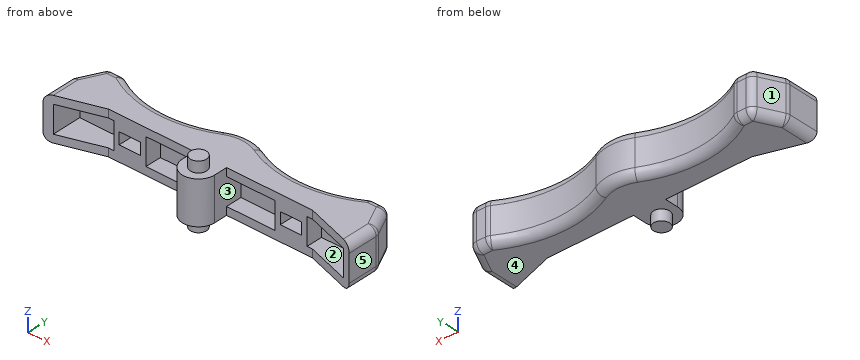
from build123d import *

# Parameters (mm, degrees)
PAD060_DEPTH            = 4
CYLINDER_R              = 1.5
CYLINDER_DEPTH          = 6
SKETCH098_W             = 9
SKETCH098_H             = 5
SKETCH098_W_2           = 4
SKETCH098_H_2           = 2.2
POCKET027_DEPTH         = 6
FILLET003_R             = 1.5
BODY091_PLACEMENT_ANGLE = 90


with BuildPart() as part:
    # Sketch097 → Pad060 (new body, symmetric)
    with BuildSketch(Plane.XZ):
        with BuildLine():
            ThreePointArc((3.619641, 7.134297), (0, 8), (-3.619641, 7.134297))
            ThreePointArc((-23, 8), (-13.423615, 5.019648), (-3.619641, 7.134297))
            Line((-23, 8), (-26, 8))
            Line((-28.5, 3), (-26, 8))
            Line((-28.5, 3), (-28.5, -3))
            Line((-19, 0), (-28.5, -3))
            Line((-3, 0), (-19, 0))
            Line((-3, 0), (-3, -2.5))
            ThreePointArc((-3, -2.5), (0, -5.5), (3, -2.5))
            Line((3, 0), (3, -2.5))
            Line((3, 0), (19, 0))
            Line((19, 0), (28.5, -3))
            Line((28.5, 3), (28.5, -3))
            Line((26, 8), (28.5, 3))
            Line((23, 8), (26, 8))
            ThreePointArc((3.619641, 7.134297), (13.423615, 5.019648), (23, 8))
        make_face()
    extrude(amount=PAD060_DEPTH, both=True)

    # Cylinder → Cylinder (join)
    with BuildSketch(Plane(origin=(0, 0, -2.5), x_dir=(1, 0, 0), z_dir=(0, -1, 0))):
        Circle(CYLINDER_R)
    cylinder = extrude(amount=CYLINDER_DEPTH)

    # Mirrored015: Cylinder across XZ
    add(cylinder.mirror(Plane.XZ))

    # Sketch098 → Pocket027 (cut)
    with BuildSketch(Plane.XY.offset(-3)):
        with Locations((-22.5, 0)):
            Rectangle(SKETCH098_W, SKETCH098_H)
        with Locations((-7.5, 0)):
            Rectangle(SKETCH098_W, SKETCH098_H)
        with Locations((-15, 0)):
            Rectangle(SKETCH098_W_2, SKETCH098_H_2)
    pocket027 = extrude(amount=POCKET027_DEPTH, mode=Mode.SUBTRACT)

    # Mirrored021: Pocket027 across YZ
    add(pocket027.mirror(Plane.YZ), mode=Mode.SUBTRACT)

    # Fillet003
    fillet003_edges = [part.edges().sort_by_distance(p)[0] for p in [
        (0, 4, 8),
        (0, -4, 8),
        (-23, 0, 8),
        (-26, 0, 8),
        (-28.5, 0, 3),
        (-28.5, 4, 0),
        (-27.25, 4, 5.5),
        (-24.5, 4, 8),
        (-13.423615, 4, 5.019648),
        (-13.423615, -4, 5.019648),
        (-24.5, -4, 8),
        (-27.25, -4, 5.5),
        (-28.5, -4, 0),
        (13.423615, -4, 5.019648),
        (13.423615, 4, 5.019648),
        (23, 0, 8),
        (26, 0, 8),
        (24.5, -4, 8),
        (24.5, 4, 8),
        (27.25, -4, 5.5),
        (28.5, -4, 0),
        (27.25, 4, 5.5),
        (28.5, 4, 0),
        (28.5, 0, 3),
    ]]
    fillet(fillet003_edges, radius=FILLET003_R)


with BuildPart() as part_1:
    # Body091 placement: moved
    add(part.part.moved(Location((40, 17, 54))).rotate(Axis((40, 17, 54), (-1, 0, 0)), BODY091_PLACEMENT_ANGLE))


solid = part_1.part
Input: part model. Units: mm. Frame: model coordinates. Face numbers are marked on the shaded views. A direction names the side the tool comes from. Give positions to 0.01 mm unless a question says otherwise; leave off trailing zeros. Loops run counter-clockwise (first coordinate to the right, second up) from the corner with the lowest first, then second, coordinate; pieces in that order, holes last. Notation, with made-up numbers: (37, 4.5) -> (69, 4.5) arc R25 ccw to (69, 28.5) -> close; hole circle Ø4 at (-11.5, -23). An arc over 180 degrees is marked (long way). Answer as a JSON object with one key per item and string values. Group by question number.
Item 1: Cut plane C-C, the plane z = 49. Return the cut outline in (x, y).
Item 2: Pin query (flat end, axial travel): P1, Ø2.5, axis at x = 16, z = 53.5, coming from the -Y side; P2, Ø5.5, axis at x = 46, z = 54.5, coming from the -Y side; P3, Ø6, axis at x = 15.5, y = 17, coming from the -Z side; P4, Ø2, axis at y = 15.5, z = 57, coming from the +X side. Return the tip coordinate at first contact, or that it passes through.
Item 3: Cut plane A-A, the plane x = 40. Return the cut outline in (y, z), and give its area (3 significant figures).
Item 4: Cut plane D-D, the plane y = 12.5. Return the cut outline in (x, z).
Item 5: Pull-direction query (Z, two-part tool) for the marked faces 3, 4 and 5; classes: released by +Z, released by -Z, zero draft, split by the parting line, or undercut.
Item 6: Line query: probe 1 along X at (y, z) = (19.5, 52.25); probe 2 along Z at (x, y) = (56.5, 19.25); probe 3 along Z at (x, y) = (38.5, 16.5). Output: solid intervals per line, ascending.
Item 7: Reachability of the marked faces 1 and 2 from +Z, -Z, +X, -X, +Y, -Y: full face, straight path, thin tool, end or side. Return the list, or none.
Checks:
{
 "1": {"outline": "circle Ø3 at (40, 14.5)"},
 "2": {"P1": "stops at y = 20", "P2": "stops at y = 17", "P3": "stops at z = 50", "P4": "stops at x = 68.5"},
 "3": {"outline": "(11.5, 50) -> (13, 50) -> (13, 48) -> (16, 48) -> (16, 50) -> (23.5, 50) arc R1.5 ccw to (25, 51.5) -> (25, 56.5) arc R1.5 ccw to (23.5, 58) -> (16, 58) -> (16, 60) -> (13, 60) -> (13, 58) -> (11.5, 58) -> close", "area": "119 mm²"},
 "4": {"outline": "(37.76, 50) -> (42.24, 50) -> (42.24, 58) -> (37.76, 58) -> close"},
 "5": {"face 3": "undercut", "face 4": "released by -Z", "face 5": "zero draft"},
 "6": {"probe 1": "x = 11.5 to 13, 22 to 28, 37 to 43, 52 to 58, 67 to 68.5", "probe 2": "z = 50 to 52.9, 55.1 to 58", "probe 3": "z = 50 to 58"},
 "7": {"face 1": "+Z, -Z, -X, +Y", "face 2": "-Y"}
}
